from build123d import *

# Parameters (mm, degrees)
SKETCH1_R               = 8
SKETCH1_R_2             = 7
BOSS_EXTRUDE1_DEPTH     = 41
CUT_EXTRUDE1_DEPTH      = 43.532340636
CUT_EXTRUDE1_DEPTH_BACK = 43.532340636
BOSS_EXTRUDE2_START     = -17
SKETCH3_R               = 7
SKETCH3_R_2             = 2.5
BOSS_EXTRUDE2_DEPTH     = 17
SKETCH4_R               = 1
CUT_EXTRUDE2_DEPTH      = 17


with BuildPart() as part:
    # Sketch1 → Boss-Extrude1 (new body)
    with BuildSketch(Plane.XY):
        Circle(SKETCH1_R)
        Circle(SKETCH1_R_2, mode=Mode.SUBTRACT)
    extrude(amount=BOSS_EXTRUDE1_DEPTH)

    # Sketch2 → Cut-Extrude1 (cut, two sides: drawn at the far end of the back side and taken through both)
    with BuildSketch(Plane(origin=(0, 0, 0), x_dir=(1, 0, 0), z_dir=(0, 1, 0)).offset(-CUT_EXTRUDE1_DEPTH_BACK)):
        with BuildLine():
            Line((-0.79375, -4), (-0.79375, -21))
            ThreePointArc((-0.79375, -21), (0, -21.79375), (0.79375, -21))
            Line((0.79375, -21), (0.79375, -4))
            ThreePointArc((0.79375, -4), (0, -3.20625), (-0.79375, -4))
        make_face()
    extrude(amount=CUT_EXTRUDE1_DEPTH + CUT_EXTRUDE1_DEPTH_BACK, mode=Mode.SUBTRACT)

    # Sketch3 → Boss-Extrude2 (add)
    with BuildSketch(Plane.XY.offset(41).offset(BOSS_EXTRUDE2_START)):
        Circle(SKETCH3_R)
        Circle(SKETCH3_R_2, mode=Mode.SUBTRACT)
    extrude(amount=BOSS_EXTRUDE2_DEPTH)

    # Sketch4 → Cut-Extrude2 (cut)
    with BuildSketch(Plane(origin=(0, 0, 0), x_dir=(1, 0, 0), z_dir=(0, 1, 0))):
        with Locations(Location((0, -26, 0), (0, 0, 90))):
            Circle(SKETCH4_R)
    extrude(amount=CUT_EXTRUDE2_DEPTH, mode=Mode.SUBTRACT)


solid = part.part
Geometry check sheet. Reference: the model listing, model coordinates, mm. A direction names the side the tool comes from. Coordinates: 2 decimals unless noted, no trailing zeros. Order: outer loops, then holes, each group sorted by start corner. A loop starts at its lowest first (then second) coordinate and runs counter-clockwise, first axis right, second up. Notation, with made-up numbers: (27.25, -2) - (41.25, -2) arc R20 cw to (41.25, 13) - close; hole circle Ø10 at (44, 0). An arc over 180 degrees is marked (long way). Answer in a Markdown table with one row per item. Add a question column.
1) Set-up check for faces 1 (the flat face through (0, -3, 24)), 2 (the cylindrical face through (-0.54, -2.44, 32.38)), 3 (the flat face through (4, -6, 0)), 4 (the cylindrical face through (0, 5, 27)), 5 (the flat face through (-0.794, 7.5, 12.4)): record each of +Z, -Z, +X, -X, +Y, -Y from which the full face is reachable in a straight line by a thin tool's end or side.
2) Release check for a two-part mould opening along X. For faces 6 (the cylindrical face through (-1.73, -7.81, 20.21)), 7 (the flat face through (-2, -2, 41)), 8 (the flat face through (0.794, -7.5, 12.6)) record: +X half, -X half, draft (parallel to the pull), parting line (faces both ways), or undercut.
3) Cross-section at A-A, the plane z = 9. Record the cut outline in (x, y).
4) Cross-section at C-C, the plane x = 0. Record the cut outline in (y, z), then the cut area to 3 significant figures.
5) Gauge pin test, flat ends, axial feed: P1, Ø1.5, axis at x = 1, z = 12.5, coming from the -Y side; P2, Ø5, axis at x = 0, y = 4, coming from the -Z side; P3, Ø1.5, axis at y = 4.5, z = 32.5, coming from the -X side. Record the tip position at first contact, or that the pin passes through.
6) Material ranges on line 1 along Y through (x, z) = (0, 37.5); line 2 along Z through (x, y) = (5.25, -1.5); line 3 along X through (y, z) = (-1.5, 23), recorded low to high. Write a range as [from, to].
7) Cross-section at B-B, the plane y = 0. Record the cut outline in (x, z), then the cut area to 3 significant figures.
8) Cross-section at D-D, the plane x = 6.25. Record the cut outline in (y, z).
Check result:
| question | item | result |
|---|---|---|
| 1 | face 1 | -Z |
| 1 | face 2 | +Z, -Z |
| 1 | face 3 | -Z, +X, -X, +Y, -Y |
| 1 | face 4 | +Y |
| 1 | face 5 | +Y, -Y |
| 2 | face 6 | parting line |
| 2 | face 7 | draft |
| 2 | face 8 | undercut |
| 3 | outline | (-0.79, -7.96) - (-0.79, -6.95) arc R7 cw to (-0.79, 6.95) - (-0.79, 7.96) arc R8 ccw to start; (0.79, -7.96) arc R8 ccw to (0.79, 7.96) - (0.79, 6.95) arc R7 cw to (0.79, -6.95) - close |
| 4 | outline | (-8, 0) - (-7, 0) - (-7, 3.21) - (-8, 3.21) - close; (-8, 21.79) - (-7, 21.79) - (-7, 24) - (-2.5, 24) - (-2.5, 41) - (-8, 41) - close; (2.5, 24) - (7, 24) - (7, 21.79) - (8, 21.79) - (8, 25) - (2.5, 25) - close; (2.5, 27) - (8, 27) - (8, 41) - (2.5, 41) - close; (7, 0) - (8, 0) - (8, 3.21) - (7, 3.21) - close |
| 4 | area | 187 mm² |
| 5 | P1 | stops at y = -7.96 |
| 5 | P2 | stops at z = 24 |
| 5 | P3 | stops at x = -7.07 |
| 6 | line 1 | y = [-8, -2.5], [2.5, 8] |
| 6 | line 2 | z = [24, 41] |
| 6 | line 3 | x = [-7.86, -6.84], [6.84, 7.86] |
| 7 | outline | (-8, 0) - (-7, 0) - (-7, 24) - (-2.5, 24) - (-2.5, 41) - (-8, 41) - close; (2.5, 24) - (7, 24) - (7, 0) - (8, 0) - (8, 41) - (2.5, 41) - close |
| 7 | area | 235 mm² |
| 8 | outline | (-4.99, 0) - (-3.15, 0) - (-3.15, 24) - (3.15, 24) - (3.15, 0) - (4.99, 0) - (4.99, 41) - (-4.99, 41) - close |
